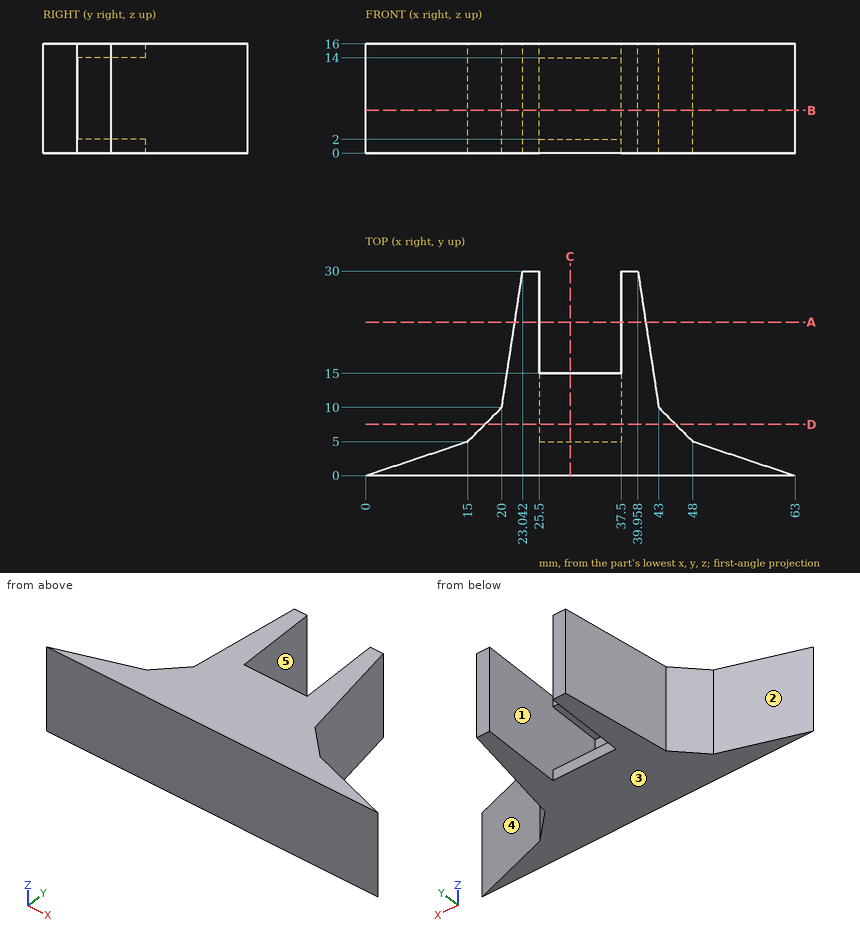
The figure shows three views and two pictorial views of one solid part (mm, origin at its lowest corner). Answer the questions. A direction names the side the tool comes from. Round coordinates to 2 decimals unless told otherwise and drop trailing zeros. Order: outer loops, then holes, each group sorted by start corner. A loop starts at its lowest first (then second) coordinate and runs counter-clockwise, first axis right, second up. Notation, with made-up numbers: (72.25, 44.25) -> (83.25, 44.25) arc R22 cw to (83.25, 76.25) -> close; hole circle Ø1 at (-23, 51). An arc over 180 degrees is marked (long way). Put each result on its own line as item: value.
Q1. Each of these flat-tipped pins is pushed along its axis until it touches: P1, Ø1, axis at x = 32, z = 1, coming from the +Y side; P2, Ø5, axis at y = 20, z = 11.5, coming from the -X side. Where does it stop, or does it pass through?
Results list:
P1: y = 15
P2: x = 21.14
Q2. Section A-A, the plane y = 22.5 is taken. Write down the section's boundary in (x, z), and give its area (3 significant figures).
Results list:
outline: (21.9, 0) -> (25.5, 0) -> (25.5, 16) -> (21.9, 16) -> close; (37.5, 0) -> (41.1, 0) -> (41.1, 16) -> (37.5, 16) -> close
area: 115 mm^2
Q3. Section B-B, the plane z = 6.25 is taken. Write down the section's boundary in (x, y), and give its area (3 significant figures).
Results list:
outline: (0, 0) -> (63, 0) -> (48, 5) -> (43, 10) -> (39.96, 30) -> (37.5, 30) -> (37.5, 5) -> (25.5, 5) -> (25.5, 30) -> (23.04, 30) -> (20, 10) -> (15, 5) -> close
area: 479 mm^2
Q4. Consider line 1 along X through (y, z) = (6, 13.75); line 2 along X through (y, z) = (19, 3.5); line 3 along Y through (x, z) = (27.5, 7.75). Determine where each line is inside the solid, lowest interval first.
Results list:
line 1: 16 to 25.5, 37.5 to 47
line 2: 21.37 to 25.5, 37.5 to 41.63
line 3: 0 to 5
Q5. Which of the six approach directions +Z, -Z, +X, -X, +Y, -Y give full straight-line access (tool end or side, diameter ignored) to the marked faces 1 and 2?
Results list:
face 1: +Y
face 2: +Z, -Z, -X, +Y
Q6. Section C-C, the plane x = 30 is taken. Write down the section's boundary in (y, z), and give its area (3 significant figures).
Results list:
outline: (0, 0) -> (15, 0) -> (15, 2) -> (5, 2) -> (5, 14) -> (15, 14) -> (15, 16) -> (0, 16) -> close
area: 120 mm^2
Q7. Determine the mould class of the marked faces 3, 4 and 5 for opening direction Z: pulls with the +Z half, pulls with the -Z half, needs draft (parallel to the pull), parting line crosses it, or undercut.
Results list:
face 3: pulls with the -Z half
face 4: needs draft
face 5: undercut
Q8. Section D-D, the plane y = 7.5 is taken. Write down the section's boundary in (x, z), and give its area (3 significant figures).
Results list:
outline: (17.5, 0) -> (45.5, 0) -> (45.5, 16) -> (17.5, 16) -> close; hole (25.5, 2) -> (37.5, 2) -> (37.5, 14) -> (25.5, 14) -> close
area: 304 mm^2
